Source: CAD feature listing. Evaluate the final solid. Frame: model axes, mm. Give positions to 0.01 mm unless a question says otherwise; leave off trailing zeros. Loops run counter-clockwise (first coordinate to the right, second up) from the corner with the lowest first, then second, coordinate; pieces in that order, holes last. Notation, with made-up numbers: M 0.5,81 L 36.5,81 A14 cw 36.5,97 Z; hole C 4.25,73.5 d5. An arc over 180 degrees is marked long. Answer in a Markdown table with one row per item.
```python
from build123d import *

# Parameters (mm, degrees)
F0_R     = 296.8625
F0_R_2   = 292.1
F1_DEPTH = 109.5375
F2_W     = 15.704696998
F2_H     = 243.4227466583
F3_DEPTH = 304.8
F5_R     = 18.5604428804
F6_DEPTH = 304.8


with BuildPart() as f1:
    # F0 (on Front) → F1 (new body)
    with BuildSketch(Plane.XZ):
        Circle(F0_R)
        Circle(F0_R_2, mode=Mode.SUBTRACT)
    extrude(amount=F1_DEPTH)

    # F2 (on Top) → F3 (cut)
    with BuildSketch(Plane.XY):
        Rectangle(F2_W, F2_H)
    extrude(amount=F3_DEPTH, mode=Mode.SUBTRACT)

    # F5 (on face) → F6 (cut)
    with BuildSketch(Plane(origin=(0, 0, 0), x_dir=(0, 1, 0), z_dir=(0.7071067812, 0, 0.7071067812))):
        with Locations((-44.45, -80.0073221326)):
            Circle(F5_R)
    extrude(amount=F6_DEPTH, mode=Mode.SUBTRACT)


solid = f1.part
```
1) Section A-A, the plane x = 89.5. Return loops of the section in (y, z).
Reply:
| item | result |
|---|---|
| outline | M -109.54,-283.05 L 0,-283.05 L 0,-278.05 L -109.54,-278.05 Z; M -109.54,278.05 L 0,278.05 L 0,283.05 L -109.54,283.05 Z |
2) Pull-direction query (Y, two-part tool) for faces 1 (the flat face through (131, 0, -262)), 2 (the cylindrical face through (261.522, -27.104, 139.037)), 3 (the flat face through (131, -109.538, -262)); classes: released by +Y, released by -Y, zero draft, split by the parting line, or undercut.
Reply:
| item | result |
|---|---|
| face 1 | released by +Y |
| face 2 | undercut |
| face 3 | released by -Y |
3) Material intervals for L1, parallel to X at y = -9, z = 3.5; L2, parallel to X at y = -47, z = 0; L3, parallel to Z at x = -160, y = -27.5, sorted ascending.
Reply:
| item | result |
|---|---|
| L1 | x = -296.84 to -292.08, 292.08 to 296.84 |
| L2 | x = -296.86 to -292.1, 292.1 to 296.86 |
| L3 | z = -250.05 to -244.38, 244.38 to 250.05 |
4) Pin query (flat end, axial travel): pin 1 Ø6 at (x, y) = (95, -84) entering from -Z; pin 2 Ø10 at (y, z) = (-79.5, 88) entering from +X; pin 3 Ø3 at (y, z) = (-33, 151.5) entering from +X. Return the tip coordinate at first contact, or that it passes through.
Reply:
| item | result |
|---|---|
| pin 1 | stops at z = -282.25 |
| pin 2 | stops at x = 285.02 |
| pin 3 | stops at x = -248.82 |
5) Section B-B, the plane y = -50. Return loops of the section in (x, z) (1 decimal), then the cut area to 3 significant figures.
Reply:
| item | result |
|---|---|
| outline | M -7.9,292 L -7.9,296.8 A296.9 ccw long 267.3,129.1 L 263.7,125.5 A292.1 cw long Z; M 7.9,292 A292.1 cw 245.8,157.7 L 249.3,161.2 A296.9 ccw 7.9,296.8 Z |
| area | 8,560 mm² |
6) Section C-C, the plane x = 0. Return loops of the section in (y, z), then the cut area to 3 significant figures.
Reply:
| item | result |
|---|---|
| outline | M -109.54,-296.86 L 0,-296.86 L 0,-292.1 L -109.54,-292.1 Z |
| area | 522 mm² |
7) Section D-D, the plane y = -98.5. Return loops of the section in (x, z) (1 decimal), then the cut area to 3 significant figures.
Reply:
| item | result |
|---|---|
| outline | M -7.9,292 L -7.9,296.8 A296.9 ccw long 7.9,296.8 L 7.9,292 A292.1 cw long Z |
| area | 8,740 mm² |
